Can you work these out from the model? Positions are in its coordinate system, mm. A direction names the side the tool comes from. Coordinates: 2 decimals unless noted, no trailing zeros. Loops run counter-clockwise (first coordinate to the right, second up) from the corner with the lowest first, then second, coordinate; pieces in that order, holes last.
Autodesk Inventor part; units mm, degrees
ref_plane "YZ Plane" through (0, 0, 0) normal (1, 0, 0) x (0, 1, 0)
ref_plane "XZ Plane" through (0, 0, 0) normal (0, 1, 0) x (-1, 0, 0)
ref_plane "XY Plane" through (0, 0, 0) normal (0, 0, 1) x (1, 0, 0)
sketch "Esquisse1" plane through (0, 0, 0) normal (0, 0, 1) x (1, 0, 0)
  circle A0 centre (0, 0) radius 8
  circle A1 centre (0, 0) radius 2.5
  point P0 (0.1533, 6)
  point P1 (-5.1195, 3.1328)
  point P2 (-5.2728, -2.8672)
  point P3 (-0.1533, -6)
  point P4 (5.1195, -3.1328)
  point P5 (5.2728, 2.8672)
  dimension "d0" = 5
  dimension "d1" = 16
  dimension "d2" = 6
  dimension "d5" = 360
extrude "Extrusion1" add sketch "Esquisse1" against normal blind 11
sketch "Esquisse2" plane through (0, 0, 0) normal (0, 0, 1) x (1, 0, 0)
  circle A0 centre (0, 0) radius 8
  point P0 (0.16, 6)
  point P1 (-5.1161, 3.1386)
  point P2 (-5.2762, -2.8614)
  point P3 (-0.16, -6)
  point P4 (5.1161, -3.1386)
  point P5 (5.2762, 2.8614)
  dimension "d9" = 6
  dimension "d12" = 360
hole "Perçage1" at (0.16, 6, 0) at (-5.1161, 3.1386, 0) at (-5.2762, -2.8614, 0) at (-0.16, -6, 0) at (5.1161, -3.1386, 0) at (5.2762, 2.8614, 0) direction (0, 0, -1) diameter 2.459 depth 8.8 tip angle 118
properties part number "moyeux_expansible"
Item 1: Suppose I cut it at C-C, the plane z = -3.75. Please give me the cut outline in (x, y).
Results are:
outline: circle Ø16 at (0, 0); hole circle Ø2.46 at (-5.28, -2.86); hole circle Ø2.46 at (-5.12, 3.14); hole circle Ø5 at (0, 0); hole circle Ø2.46 at (-0.16, -6); hole circle Ø2.46 at (0.16, 6); hole circle Ø2.46 at (5.12, -3.14); hole circle Ø2.46 at (5.28, 2.86)
Item 2: On a 3-axis mill with a long thin cutter (end or side, diameter ignored), from which of +Z, -Z, +X, -X, +Y, -Y can I reach the whole of each face in a straight line? I mean faces 1 (the face through (-0.54, -2.44, -5.42)), 2 (the face through (4.057, 3.021, -4.462)). Say none if no direction works.
Results are:
face 1: +Z, -Z
face 2: +Z
Item 3: I need wall thicknesses on line 1 along Y through (x, z) = (0.25, -1); line 2 along X through (y, z) = (2.75, -0.5); line 3 along Y through (x, z) = (5, -0.75) (3 decimals). Which ranges of each line are inside material? Lowest first, please.
Results are:
line 1: y = -8 to -7.16, -4.84 to -2.49, 2.49 to 4.77, 7.23 to 8
line 2: x = -7.51 to -6.28, -3.95 to 4.05, 6.5 to 7.51
line 3: y = -6.245 to -4.363, -1.915 to 1.663, 4.059 to 6.245
Item 4: We'd pull the mould along Y, two halves only. Please class faces 3 (the face through (3.897, -2.979, -4.462)), 4 (the face through (2, 2, 0)), 5 (the face through (-1.73, -7.81, -5.42)): +Y half, -Y half, draft (parallel to the pull), parting line (faces both ways), or undercut.
Results are:
face 3: undercut
face 4: draft
face 5: parting line
Item 5: Suppose I cut it at A-A, the plane y = 0. Please give me the cut outline in (x, z), plus the area to 3 significant figures.
Results are:
outline: (-8, -11) - (-2.5, -11) - (-2.5, 0) - (-8, 0) - close; (2.5, -11) - (8, -11) - (8, 0) - (2.5, 0) - close
area: 121 mm2
Item 6: Suppose I cut it at D-D, the plane x = -2.75. Please give me the cut outline in (y, z).
Results are:
outline: (-7.51, -11) - (7.51, -11) - (7.51, 0) - (-7.51, 0) - close
Item 7: Suppose I cut it at B-B, the plane x = 1.75. Please give me the cut outline in (y, z).
Results are:
outline: (-7.81, -11) - (-1.79, -11) - (-1.79, 0) - (-7.81, 0) - close; (1.79, -11) - (7.81, -11) - (7.81, 0) - (1.79, 0) - close
Item 8: I'm going to push flat-ended pins straight in: P1, Ø1, axis at x = -4.5, z = -7.5, coming from the +Y side; P2, Ø1.5, axis at x = 5.12, y = -3.14, coming from the +Z side; P3, Ø6, axis at x = 5.5, z = -7, coming from the -Y side. Where does each tip first touch, or does it pass through?
Results are:
P1: stops at y = 6.93
P2: stops at z = -9.09
P3: stops at y = -7.6
